Autodesk Inventor part; units mm, degrees
ref_plane "YZ Plane" through (0, 0, 0) normal (1, 0, 0) x (0, 1, 0)
ref_plane "XZ Plane" through (0, 0, 0) normal (0, 1, 0) x (-1, 0, 0)
ref_plane "XY Plane" through (0, 0, 0) normal (0, 0, 1) x (1, 0, 0)
sketch "Sketch1" plane through (0, 0, 0) normal (1, 0, 0) x (0, 1, 0)
  line L0 (0, 0) -> (0, -17)
  circle A0 centre (0, 0) radius 1.6
  circle A1 centre (0, -17) radius 1.6
  circle A2 centre (0, 0) radius 3.25
  circle A3 centre (0, -17) radius 3.25
  circle A4 centre (0, -8.5) radius 6.5
  line L1 (3.25, 0) -> (3.25, -17)
  line L2 (-3.25, 0) -> (-3.25, -17)
  point P0 (3.25, -14.1292)
  point P1 (3.25, -2.8708)
  point P2 (-3.25, -2.8708)
  point P3 (-3.25, -14.1292)
  dimension "d3" = 6.5
  dimension "d4" = 6.5
  dimension "d0" = 17
  dimension "d1" = 3.2
  dimension "d2" = 3.2
  dimension "d5" = 13
extrude "Extrusion1" add sketch "Sketch1" along normal blind 2
sketch "Sketch2" plane through (2, 0, 0) normal (1, 0, 0) x (0, 0, -1)
  arc A0 (14.1292, 3.25) -> (2.8708, 3.25) centre (8.5, 0) ccw
  circle A1 centre (8.5, 0) radius 6.5
  circle A2 centre (8.5, 0) radius 3.95
  point P0 (0, 0)
  point P1 (2.8708, 3.25)
  point P2 (14.1292, 3.25)
  dimension "d8" = 7.9
extrude "Extrusion2" add sketch "Sketch2" along normal blind 7
sketch "Sketch3" plane through (2, 0, 0) normal (1, 0, 0) x (0, 0, -1)
  circle A0 centre (0, 0) radius 3
  circle A1 centre (17, 0) radius 1.6
  circle A2 centre (17, 0) radius 3
  dimension "d11" = 6
  dimension "d12" = 6
extrude "Extrusion3" cut sketch "Sketch3" along normal through all contours A0 | A1 | A2
sketch "Sketch4" plane through (0, 0, 0) normal (-1, 0, 0) x (0, 0, 1)
  circle A0 centre (-8.5, 0) radius 3.95
  line L0 (-8.5, 0) -> (-8.5, 3.95)
  line L1 (-5.7, 6.45) -> (-11.3, 6.45)
  line L2 (-11.3, 6.45) -> (-11.3, 1.45)
  line L3 (-11.3, 1.45) -> (-5.7, 1.45)
  line L4 (-5.7, 1.45) -> (-5.7, 6.45)
  line L5 (-5.7, 6.45) -> (-11.3, 1.45) construction
  line L6 (-11.3, 6.45) -> (-5.7, 1.45) construction
  line L7 (-11.3, 3.95) -> (-5.7, 3.95)
  line L8 (-12.45, -7.9907) -> (-4.55, -7.9907)
  line L9 (-4.55, -7.9907) -> (-4.55, 7.9907)
  line L10 (-4.55, 7.9907) -> (-12.45, 7.9907)
  line L11 (-12.45, 7.9907) -> (-12.45, -7.9907)
  line L12 (-12.45, -7.9907) -> (-4.55, 7.9907) construction
  line L13 (-4.55, -7.9907) -> (-12.45, 7.9907) construction
  arc A1 (-2.2941, 1.9331) -> (-14.7059, 1.9331) centre (-8.5, 0) ccw
  line L14 (-4.55, 5.1621) -> (-12.45, 5.1621)
  point P0 (0, 0)
  point P1 (-5.7, 5.1621)
  point P2 (-5.7, 2.7861)
  point P3 (-4.55, 0)
  dimension "d15" = 5.6
  dimension "d16" = 5
extrude "Extrusion4" add sketch "Sketch4" against normal blind 9 contours A0 L4 L14 L9 | A1 L4 L1 L2 L11 L10 L9 | L14 L4 A1 | A1 L2 L14 | A1 L1 L4 | L4 L14 L2 A1 L1 | L2 L1 A1 | L1 A1
sketch "Sketch5" plane through (9, 0, 0) normal (1, 0, 0) x (0, 0, -1)
  circle A0 centre (8.5, 0) radius 3.95
  line L0 (8.5, 0) -> (8.5, 3.95)
  line L1 (5.7, 1.45) -> (11.3, 1.45)
  line L2 (11.3, 1.45) -> (11.3, 6.45)
  line L3 (11.3, 6.45) -> (5.7, 6.45)
  line L4 (5.7, 6.45) -> (5.7, 1.45)
  line L5 (5.7, 1.45) -> (11.3, 6.45) construction
  line L6 (11.3, 1.45) -> (5.7, 6.45) construction
  line L7 (8.5, 3.95) -> (5.7, 3.95)
  line L8 (5.7, 3.95) -> (11.3, 3.95)
  point P0 (0, 0)
  dimension "d19" = 5.6
  dimension "d20" = 5
extrude "Extrusion5" cut sketch "Sketch5" against normal blind 6 contours L7 L4 L3 L2 L8
sketch "Sketch6" plane through (0, 7.9907, -4.55) normal (0, 1, 0) x (1, 0, 0)
  point P0 (0, -4.55)
sketch "Sketch7" plane through (0, 7.9907, -4.55) normal (0, 1, 0) x (1, 0, 0)
  line L0 (9, 3.95) -> (3, 3.95)
  line L1 (3.8147, 3.95) -> (6.916, 3.95) construction
  line L2 (3.8147, 2.35) -> (6.916, 2.35)
  line L3 (6.916, 5.55) -> (3.8147, 5.55)
  arc A0 (3.8147, 5.55) -> (3.8147, 2.35) centre (3.8147, 3.95) ccw
  arc A1 (6.916, 2.35) -> (6.916, 5.55) centre (6.916, 3.95) ccw
  point P0 (0, -4.55)
  point P1 (5.3654, 3.95)
  dimension "d23" = 3.2
sketch "Sketch8" plane through (9, 3.95, -8.5) normal (0, 1, 0) x (1, 0, 0)
  line L0 (0, 0) -> (0, -2.8)
  line L1 (-7, -3.95) -> (-7, 3.95)
  line L2 (0, -2.8) -> (-7, -2.8)
  line L3 (-7, -2.8) -> (-7, 2.7358)
  line L4 (0, -2.8) -> (-7, -2.8)
  line L5 (-7, -2.8) -> (-7, 2.8)
  line L6 (-7, 2.8) -> (0, 2.8)
  line L7 (0, 2.8) -> (0, -2.8)
  point P0 (-9, -8.5)
  dimension "d28" = 5.6
sketch "Sketch9" plane through (9, 0, 0) normal (1, 0, 0) x (0, 0, -1)
  line L0 (5.7, 3.95) -> (5.7, 6.45)
  line L1 (5.7, 6.45) -> (11.3, 6.45)
  line L2 (11.3, 6.45) -> (11.3, 7.2)
  line L3 (11.3, 7.2) -> (5.7, 7.2)
  line L4 (5.7, 7.2) -> (5.7, 6.45)
  point P0 (0, 0)
  dimension "d29" = 0.75
extrude "Extrusion8" cut sketch "Sketch9" against normal blind 6
sketch "Sketch10" plane through (9, 0, 0) normal (1, 0, 0) x (0, 0, -1)
  line L0 (11.3, 7.2) -> (11.3, 3.95)
  line L1 (5.7, 3.95) -> (5.7, 7.2)
  line L2 (11.3, 3.95) -> (5.7, 3.95)
  line L3 (5.7, 3.95) -> (5.7, 4.7)
  line L4 (5.7, 4.7) -> (11.3, 4.7)
  line L5 (11.3, 4.7) -> (11.3, 3.95)
  point P0 (0, 0)
  dimension "d32" = 0.75
extrude "Extrusion9" add sketch "Sketch10" against normal blind 6
sketch "Sketch11" plane through (0, 7.9907, -4.55) normal (0, 1, 0) x (1, 0, 0)
  line L0 (0, -1.6792) -> (0, 0)
  line L1 (9, 7.9) -> (9, 10.1559)
  line L2 (0, 0) -> (9, 0)
  line L3 (9, 0) -> (9, 7.9)
  line L4 (9, 7.9) -> (0, 7.9)
  line L5 (0, 7.9) -> (0, 0)
  point P0 (0, -4.55)
extrude "Extrusion11" add sketch "Sketch11" along normal blind 1.5
extrude "Extrusion12" cut sketch "Sketch7" along normal mid plane 10
fillet "Fillet1" radius 1 2 edges at (4.5, 9.4907, -4.55) (4.5, 9.4907, -12.45)
sketch "Sketch12" plane through (2, 0, 0) normal (1, 0, 0) x (0, 0, -1)
  circle A0 centre (0, 0) radius 1.6
  circle A1 centre (0, 0) radius 2.1992
  circle A2 centre (17, 0) radius 1.6
  circle A3 centre (17, 0) radius 2.2664
extrude "Extrusion13" add sketch "Sketch12" against normal blind 2 contours A0 | A1 | A2 | A3
sketch "Sketch13" plane through (2, 0, 0) normal (1, 0, 0) x (0, 0, -1)
  circle A0 centre (0, 0) radius 1.475
  arc A1 (17, -3.25) -> (17, 3.25) centre (17, 0) ccw
  circle A2 centre (17, 0) radius 1.475
  dimension "d44" = 2.95
  dimension "d45" = 2.95
extrude "Extrusion14" cut sketch "Sketch13" against normal blind 2
sketch "Sketch14" plane through (2, 0, -8.5) normal (1, 0, 0) x (0, 0, -1)
  circle A0 centre (0, 0) radius 3.95
  point P0 (-8.5, 0)
extrude "Extrusion15" cut sketch "Sketch14" against normal blind 10
sketch "Sketch15" plane through (2, 0, 0) normal (1, 0, 0) x (0, 0, -1)
  point P0 (0, 0)
properties part number "acople2"
Source: CAD feature listing. Evaluate the final solid. Frame: model axes, mm. A direction names the side the tool comes from. Give positions to 0.01 mm unless a question says otherwise; leave off trailing zeros. Write each loop counter-clockwise with the first axis right and the second up, starting at its lowest first coordinate (ties: lowest second). Pieces come first, ordered by that corner, then holes. Notation, with made-up numbers: (62.25, 63.25) -> (111.25, 63.25) arc R24 ccw to (111.25, 102.25) -> close; hole circle Ø2 at (86.5, 70). An arc over 180 degrees is marked (long way). Return JSON: item names as keys, results as strings. Group by question number.
1. Section A-A, the plane z = -8.5. Output: boundary loops of the cut face in (x, y), then the cut area to 3 significant figures.
2. Section C-C, the plane y = -3. Output: boundary loops of the cut face in (x, z), then the cut area to 3 significant figures.
3. Access query for faces 5 (the face through (5, 0, -3)), 6 (the face through (2.215, 6.51, -8.465)), 7 (the face through (3, 6, -11)). Directions: +Z, -Z, +X, -X, +Y, -Y. A direction counts if a zero-diameter tool reaches every point of the face in a straight line with its end or side. Return the directions, or none.
4. Section B-B, the plane y = 0. Output: boundary loops of the cut face in (x, z) (3 decimals), then the cut area to 3 significant figures.
5. Section D-D, the plane z = -12. Output: boundary loops of the cut face in (x, y).
6. Pin query (flat end, axial travel): pin 1 Ø2 at (x, z) = (1, -15.5) entering from -Y; pin 2 Ø2 at (x, z) = (0.5, -1) entering from +Y; pin 3 Ø4 at (x, y) = (1.5, 3) entering from -Z; pin 4 Ø2 at (x, z) = (1, -12) entering from +Y. Return the tip coordinate at first contact, or that it passes through.
7. Material intervals for line 1 (Z direction, x = 5, y = 8.5); line 2 (Y direction, x = 1.55, z = 0) (3 decimals); line 3 (Z direction, x = 4.5, y = 6.75), sorted ascending. Write a range as from..to.
8. Mould query, pull axis Y, two halves, no side actions, for faces 1 (the face through (5.451, 4.303, -13.372)), 2 (the face through (5, 0, -14)), 3 (the face through (5, 7, -12.45)), 4 (the face through (4.4, -6.5, -8.6)). Classes: +Y half, -Y half, draft (parallel to the pull), parting line (faces both ways), or undercut.
Determined:
{
 "1": {"outline": "(0, -6.5) -> (9, -6.5) -> (9, -3.95) -> (0, -3.95) -> close; (0, 3.95) -> (2.21, 3.95) -> (2.21, 9.49) -> (0, 9.49) -> close; (8.52, 3.95) -> (9, 3.95) -> (9, 4.7) -> (8.52, 4.7) -> close; (8.52, 7.2) -> (9, 7.2) -> (9, 9.49) -> (8.52, 9.49) -> close", "area": "36.7 mm2"},
 "2": {"outline": "(0, -18.25) -> (2, -18.25) -> (2, -14.27) -> (9, -14.27) -> (9, -11.07) -> (0, -11.07) -> close; (0, -5.93) -> (9, -5.93) -> (9, -2.73) -> (2, -2.73) -> (2, 1.25) -> (0, 1.25) -> close", "area": "73.5 mm2"},
 "3": {"face 5": "+Z, +X", "face 6": "+Y", "face 7": "+X"},
 "4": {"outline": "(0, -20.25) -> (2, -20.25) -> (2, -18.475) -> (0, -18.475) -> close; (0, -15.525) -> (2, -15.525) -> (2, -14) -> (9, -14) -> (9, -12.45) -> (0, -12.45) -> close; (0, -4.55) -> (9, -4.55) -> (9, -3) -> (2, -3) -> (2, -1.475) -> (0, -1.475) -> close; (0, 1.475) -> (2, 1.475) -> (2, 3.25) -> (0, 3.25) -> close", "area": "41.1 mm2"},
 "5": {"outline": "(0, -5.48) -> (9, -5.48) -> (9, -1.83) -> (0, -1.83) -> close; (0, 1.83) -> (9, 1.83) -> (9, 9.33) -> (0, 9.33) -> close"},
 "6": {"pin 1": "stops at y = -3.25", "pin 2": "stops at y = 3.25", "pin 3": "stops at z = -20.09", "pin 4": "stops at y = 9.49"},
 "7": {"line 1": "z = -12.45..-10.1, -6.9..-4.55", "line 2": "y = -3.25..-1.475, 1.475..3.25", "line 3": "z = -12.45..-11.3, -5.7..-4.55"},
 "8": {"face 1": "+Y half", "face 2": "undercut", "face 3": "draft", "face 4": "-Y half"}
}
